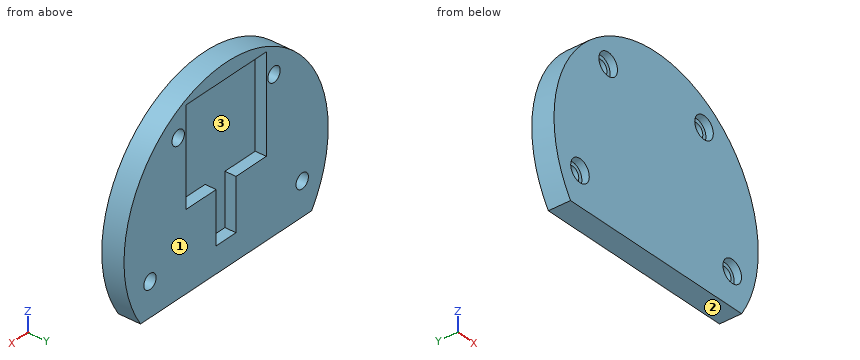
```python
from build123d import *

# Parameters (mm, degrees)
SKETCH_1_R          = 16.5
EXTRUDE_1_DEPTH     = 3
SKETCH_2_W          = 13
SKETCH_2_H          = 13
CUT_EXTRUDE_1_DEPTH = 1.5
SKETCH_3_W          = 3.2
SKETCH_3_H          = 7
CUT_EXTRUDE_2_DEPTH = 1.5
SKETCH_4_R          = 1.5
SKETCH_4_R_2        = 1
CUT_EXTRUDE_3_DEPTH = 1
SKETCH_4_2_R        = 1
CUT_EXTRUDE_4_DEPTH = 24.526580712
SKETCH_5_W          = 27.658633372
SKETCH_5_H          = 9.051760597
CUT_EXTRUDE_5_DEPTH = 24.526580712


with BuildPart() as part:
    # 草图1 → 凸台-拉伸1 (new body)
    with BuildSketch(Plane(origin=(0, 0, 0), x_dir=(1, 0, 0), z_dir=(0, 1, 0))):
        with Locations(Location((0, 0, 0), (0, 0, 270))):
            Circle(SKETCH_1_R)
    extrude(amount=EXTRUDE_1_DEPTH)

    # 草图2 → 切除-拉伸1 (cut)
    with BuildSketch(Plane(origin=(0, 3, 0), x_dir=(1, 0, 0), z_dir=(0, 1, 0))):
        with Locations((0, -8)):
            Rectangle(SKETCH_2_W, SKETCH_2_H)
    extrude(amount=-CUT_EXTRUDE_1_DEPTH, mode=Mode.SUBTRACT)

    # 草图3 → 切除-拉伸2 (cut)
    with BuildSketch(Plane(origin=(0, 3, 0), x_dir=(1, 0, 0), z_dir=(0, 1, 0))):
        with Locations((0, 2)):
            Rectangle(SKETCH_3_W, SKETCH_3_H)
    extrude(amount=-CUT_EXTRUDE_2_DEPTH, mode=Mode.SUBTRACT)

    # 草图4 → 切除-拉伸3 (cut)
    # profile 1 of 4: a face of its own
    with BuildSketch(Plane.XZ):
        with Locations(Location((7.743281891, 11.058552598, 0), (0, 0, 270))):
            Circle(SKETCH_4_R)
        with Locations(Location((7.743281891, 11.058552598, 0), (0, 0, 270))):
            Circle(SKETCH_4_R_2, mode=Mode.SUBTRACT)
    # profile 2 of 4: a face of its own
    with BuildSketch(Plane.XZ):
        with Locations(Location((-7.743281891, 11.058552598, 0), (0, 0, 270))):
            Circle(SKETCH_4_R)
        with Locations(Location((-7.743281891, 11.058552598, 0), (0, 0, 270))):
            Circle(SKETCH_4_R_2, mode=Mode.SUBTRACT)
    # profile 3 of 4: a face of its own
    with BuildSketch(Plane.XZ):
        with Locations(Location((-12.3, -4.5, 0), (0, 0, 270))):
            Circle(SKETCH_4_R)
        with Locations(Location((-12.3, -4.5, 0), (0, 0, 270))):
            Circle(SKETCH_4_R_2, mode=Mode.SUBTRACT)
    # profile 4 of 4: a face of its own
    with BuildSketch(Plane.XZ):
        with Locations(Location((12.3, -4.5, 0), (0, 0, 270))):
            Circle(SKETCH_4_R)
        with Locations(Location((12.3, -4.5, 0), (0, 0, 270))):
            Circle(SKETCH_4_R_2, mode=Mode.SUBTRACT)
    extrude(amount=-CUT_EXTRUDE_3_DEPTH, mode=Mode.SUBTRACT)

    # 草图4<2> → 切除-拉伸4 (cut, through all)
    with BuildSketch(Plane.XZ):
        with Locations(Location((7.743281891, 11.058552598, 0), (0, 0, 270))):
            Circle(SKETCH_4_2_R)
        with Locations(Location((-7.743281891, 11.058552598, 0), (0, 0, 270))):
            Circle(SKETCH_4_2_R)
        with Locations(Location((-12.3, -4.5, 0), (0, 0, 270))):
            Circle(SKETCH_4_2_R)
        with Locations(Location((12.3, -4.5, 0), (0, 0, 270))):
            Circle(SKETCH_4_2_R)
    extrude(amount=-CUT_EXTRUDE_4_DEPTH, mode=Mode.SUBTRACT)

    # 草图5 → 切除-拉伸5 (cut, through all)
    with BuildSketch(Plane(origin=(0, 3, 0), x_dir=(1, 0, 0), z_dir=(0, 1, 0))):
        with Locations((0, 13.525880299)):
            Rectangle(SKETCH_5_W, SKETCH_5_H)
    extrude(amount=-CUT_EXTRUDE_5_DEPTH, mode=Mode.SUBTRACT)


solid = part.part
```
For this review, take the finished solid that the model builds, in its own axes (mm). Face numbers are marked on the shaded views. Round coordinates to 2 decimals unless told otherwise and drop trailing zeros. Write each loop counter-clockwise with the first axis right and the second up, starting at its lowest first coordinate (ties: lowest second). Pieces come first, ordered by that corner, then holes. Notation, with made-up numbers: (54.5, -10) - (82.5, -10) arc R29 cw to (82.5, 12) - close; hole circle Ø8 at (42, 20). An arc over 180 degrees is marked (long way). Answer as a JSON object with one key per item and string values.
1. We need section B-B on y = 2.35. Give the boundary of the cut face in (x, z).
Response values:
{"outline": "(-13.83, -9) - (13.83, -9) arc R16.5 ccw (long way) to start; hole circle Ø2 at (-12.3, -4.5); hole circle Ø2 at (-7.74, 11.06); hole (-6.5, 1.5) - (-1.6, 1.5) - (-1.6, -5.5) - (1.6, -5.5) - (1.6, 1.5) - (6.5, 1.5) - (6.5, 14.5) - (-6.5, 14.5) - close; hole circle Ø2 at (7.74, 11.06); hole circle Ø2 at (12.3, -4.5)"}
2. We need section D-D on x = 0. Give the boundary of the cut face in (y, z), then the cut area to 3 significant figures.
Response values:
{"outline": "(0, -9) - (3, -9) - (3, -5.5) - (1.5, -5.5) - (1.5, 14.5) - (3, 14.5) - (3, 16.5) - (0, 16.5) - close", "area": "46.5 mm2"}
3. We need section C-C on x = -12.3. Give the boundary of the cut face in (y, z).
Response values:
{"outline": "(0, -9) - (3, -9) - (3, -5.5) - (1, -5.5) - (1, -6) - (0, -6) - close; (0, -3) - (1, -3) - (1, -3.5) - (3, -3.5) - (3, 11) - (0, 11) - close"}
4. For pin 1 Ø1 at (y, z) = (0.5, -3) entering from -X; pin 2 Ø1 at (y, z) = (2, -2.5) entering from +X; pin 3 Ø1.5 at (y, z) = (1, -4) entering from -X; pin 4 Ø1.6 at (x, z) = (-12.3, -4.5) entering from -Y, all flat-tipped, find the tip position at first contact; note any pin that passes through.
Response values:
{"pin 1": "stops at x = -16.31", "pin 2": "stops at x = 16.38", "pin 3": "stops at x = -16.18", "pin 4": "passes through"}
5. We need section A-A on z = -4.5. Give the boundary of the cut face in (x, y).
Response values:
{"outline": "(-15.87, 0) - (-13.8, 0) - (-13.8, 1) - (-13.3, 1) - (-13.3, 3) - (-15.87, 3) - close; (-11.3, 1) - (-10.8, 1) - (-10.8, 0) - (10.8, 0) - (10.8, 1) - (11.3, 1) - (11.3, 3) - (1.6, 3) - (1.6, 1.5) - (-1.6, 1.5) - (-1.6, 3) - (-11.3, 3) - close; (13.3, 1) - (13.8, 1) - (13.8, 0) - (15.87, 0) - (15.87, 3) - (13.3, 3) - close"}
6. Draft analysis for pull direction Z (two halves, no side actions). For the marked faces 1, 2 and 3, state which applies: +Z half, -Z half, draft (parallel to the pull), parting line (faces both ways), or undercut.
Response values:
{"face 1": "draft", "face 2": "-Z half", "face 3": "undercut"}
7. To check wall thickness, follow line 1 along X through (y, z) = (2.3, -4.25); line 2 along Y through (x, z) = (9, 11.5); line 3 along Y through (x, z) = (3, 2.75). State the ranges of each line that lie inside material, in increasing order.
Response values:
{"line 1": "x = -15.94 to -13.27, -11.33 to -1.6, 1.6 to 11.33, 13.27 to 15.94", "line 2": "y = 1 to 3", "line 3": "y = 0 to 1.5"}
